Build history of the part. All positions in model axes, mm. Face numbers are marked on the shaded views. A direction names the side the tool comes from. Round coordinates to 2 decimals unless told otherwise and drop trailing zeros. Loops run counter-clockwise (first coordinate to the right, second up) from the corner with the lowest first, then second, coordinate; pieces in that order, holes last. Notation, with made-up numbers: M 2.25,-24 L 33.25,-24 A22 cw 33.25,-2 Z; hole C 12.5,87.25 d7. An arc over 180 degrees is marked long. Use one line per item in the form item = value. Start each with the question number.
```python
from build123d import *

# Parameters (mm, degrees)
SKETCH1_R           = 5.55
SKETCH1_R_2         = 2.55
BOSS_EXTRUDE1_DEPTH = 5
SKETCH2_R           = 8.55
BOSS_EXTRUDE2_DEPTH = 2


with BuildPart() as part:
    # Sketch1 → Boss-Extrude1 (new body)
    with BuildSketch(Plane.XY):
        Circle(SKETCH1_R)
        Circle(SKETCH1_R_2, mode=Mode.SUBTRACT)
    extrude(amount=-BOSS_EXTRUDE1_DEPTH)

    # Sketch2 → Boss-Extrude2 (add)
    with BuildSketch(Plane.XY):
        Circle(SKETCH2_R)
    extrude(amount=BOSS_EXTRUDE2_DEPTH)


solid = part.part
```
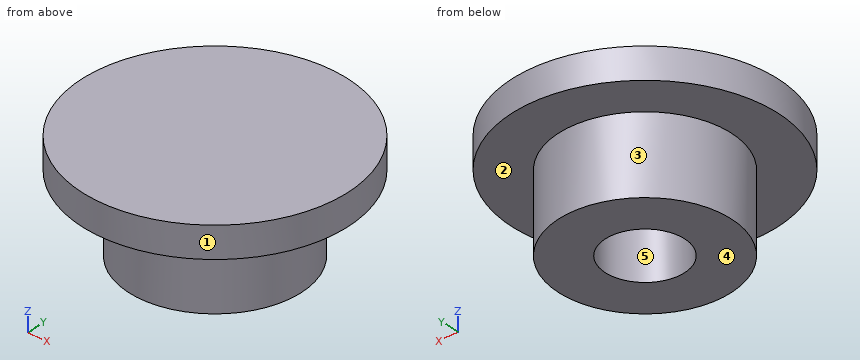
Q1. Pull direction X, two halves, no side cores. Call the marked faces 3, 4 and 5: pulls with the +X half, pulls with the -X half, needs draft (parallel to the pull), parting line crosses it, or undercut.
Q2. Tool access for the marked faces 1 and 2: list every direction of +Z, -Z, +X, -X, +Y, -Y with a clear straight run to the whole face (end or side of a thin tool).
Q3. Saw through at C-C (z = -2.25). Give the cut face in (x, y).
Q4. Wall check: probe 1 along Y at (x, z) = (0, -1.85); probe 2 along Z at (x, y) = (1, -0.5); probe 3 along X at (y, z) = (2.25, -0.5). Give the ranges that are in metal, low to high.
Q5. Drop flat-ended pins along their axis: P1, Ø6.5, axis at x = 0, y = 0, coming from the -Z side; P2, Ø4, axis at x = 3, z = -3, coming from the -Y side; P3, Ø2.5, axis at x = 0, y = -0.5, coming from the -Z side; P4, Ø1, axis at x = 1.5, z = 1, coming from the +Y side. Give the stop position or say it passes through.
Q6. Saw through at A-A (x = 0). Give the cut face in (y, z).
Q7. Saw through at D-D (x = -3.5). Give the cut face in (y, z), and give its area (3 significant figures).
Filled in:
q1.face_3 = parting line crosses it
q1.face_4 = needs draft
q1.face_5 = undercut
q2.face_1 = +Z, -Z
q2.face_2 = -Z
q3.outline = C 0,0 d11.1; hole C 0,0 d5.1
q4.probe_1 = -5.55 to -2.55, 2.55 to 5.55
q4.probe_2 = 0 to 2
q4.probe_3 = -5.07 to -1.2, 1.2 to 5.07
q5.P1 = -5
q5.P2 = -5.46
q5.P3 = 0
q5.P4 = 8.49
q6.outline = M -8.55,0 L -5.55,0 L -5.55,-5 L -2.55,-5 L -2.55,0 L 2.55,0 L 2.55,-5 L 5.55,-5 L 5.55,0 L 8.55,0 L 8.55,2 L -8.55,2 Z
q7.outline = M -7.8,0 L -4.31,0 L -4.31,-5 L 4.31,-5 L 4.31,0 L 7.8,0 L 7.8,2 L -7.8,2 Z
q7.area = 74.3 mm²
